Read the model definition and answer for the solid it produces. Units are mm, in the model's axes. A direction names the side the tool comes from. Coordinates: 2 decimals unless noted, no trailing zeros. Loops run counter-clockwise (first coordinate to the right, second up) from the corner with the lowest first, then second, coordinate; pieces in that order, holes last. Notation, with made-up numbers: M -30,55 L 9,55 A22 ccw 9,81 Z; hole C 21.5,41.25 d7. An arc over 180 degrees is marked long. One line per item, written item: value. Start each with the question number.
1. Flat-ended cylindrical pins translate along their axes: pin 1 (18.5 mm diameter, centred on x = 53.975, y = 0, fed in from -Z); pin 2 (1.3 mm diameter, centred on x = 16.5, z = 11.5, fed in from +Y); pin 3 (1.5 mm diameter, centred on x = 14.5, z = 6.5, fed in from -Y); pin 4 (2 mm diameter, centred on x = 15, z = 27.5, fed in from -Y). Find the tip coordinate at first contact, or state that the pin passes through.
2. The part is cut by section B-B (x = 55). Write down the section's boundary in (y, z), then the cut area to 3 significant figures.
3. Consider probe 1 along Y at (x, z) = (0, 22) (1 decimal); probe 2 along X at (y, z) = (0, 29) (1 decimal); probe 3 along Z at (x, y) = (43.5, 9.5). Determine where each line is inside the solid, lowest interval first.
4. Determine the mould class of faces 3 (the face through (22, 0, 0)), 4 (the face through (73.02, -0.42, 7.78)), 5 (the face through (-14.277, -0.559, 19.835)), 6 (the face through (-28.547, 1.256, 22.311)) for opening direction X: +X half, -X half, draft (parallel to the pull), parting line (faces both ways), or undercut.
5. The part is cut by section A-A (z = 10). State how many separate pieces and enclosed holes the cut face has, then the cut area to 3 significant figures.
6. For faces 1 (the face through (16, 4.826, 20)), 2 (the face through (29.252, -23.636, 7.776)), determine the directions among +Z, -Z, +X, -X, +Y, -Y from which every point of the face is accessible in a straight line to the end or side of a thin tool.
```python
from build123d import *

# Parameters (mm, degrees)
F0_R     = 10.16
F1_DEPTH = 15.7734
F3_DEPTH = 40.2336
F4_R     = 3.302


with BuildPart() as f1:
    # F0 (on Top) → F1 (new body)
    with BuildSketch(Plane.XY):
        with BuildLine():
            ThreePointArc((5.2118165849, 28.0956863751), (21.9710978778, 18.270234893), (28.575, 0))
            ThreePointArc((28.575, 0), (21.9710977085, -18.2702350965), (5.2118160642, -28.0956864716))
            Line((5.2118160642, -28.0956864716), (53.975, -19.05))
            ThreePointArc((53.975, -19.05), (34.925, 0), (53.975, 19.05))
            Line((53.975, 19.05), (5.2118165849, 28.0956863751))
        make_face()
        with BuildLine():
            ThreePointArc((73.025, 0), (67.4453841816, 13.4703841816), (53.975, 19.05))
            ThreePointArc((53.975, 19.05), (34.925, 0), (53.975, -19.05))
            ThreePointArc((53.975, -19.05), (67.4453841816, -13.4703841816), (73.025, 0))
        make_face()
        with Locations((53.975, 0)):
            Circle(F0_R, mode=Mode.SUBTRACT)
    extrude(amount=F1_DEPTH)

    # F2 (on face) → F3 (join)
    with BuildSketch(Plane.XY):
        with BuildLine():
            ThreePointArc((5.2118165849, 28.0956863751), (-28.575, 2.648e-07), (5.2118160642, -28.0956864716))
            ThreePointArc((5.2118160642, -28.0956864716), (21.9710977085, -18.2702350965), (28.575, 0))
            ThreePointArc((28.575, 0), (21.9710978778, 18.270234893), (5.2118165849, 28.0956863751))
        make_face()
        with BuildLine():
            Line((17.6895648793, -4.826), (13.4477648793, -4.826))
            ThreePointArc((13.4477648793, -4.826), (-14.2875, 0), (13.4477648793, 4.826))
            Line((13.4477648793, 4.826), (17.6895648793, 4.826))
            Line((17.6895648793, 4.826), (17.6895648793, -4.826))
        make_face(mode=Mode.SUBTRACT)
    extrude(amount=F3_DEPTH)

    # F4
    f4_edges = [f1.edges().sort_by_distance(p)[0] for p in [
        (-5.211816, 28.095686, 40.2336),
    ]]
    fillet(f4_edges, radius=F4_R)


solid = f1.part
```
Answer block:
1. pin 1: passes through
1. pin 2: stops at y = 26.12
1. pin 3: stops at y = -26.51
1. pin 4: stops at y = -24.91
2. outline: M -19.02,0 L -10.11,0 L -10.11,15.77 L -19.02,15.77 Z; M 10.11,0 L 19.02,0 L 19.02,15.77 L 10.11,15.77 Z
2. area: 281 mm2
3. probe 1: y = -28.6 to -14.3, 14.3 to 28.6
3. probe 2: x = -28.6 to -14.3, 17.7 to 28.6
3. probe 3: z = 0 to 15.77
4. face 3: draft
4. face 4: +X half
4. face 5: undercut
4. face 6: parting line
5. separate pieces: 1
5. enclosed holes: 2
5. area: 3,450 mm2
6. face 1: +Z, -Z
6. face 2: +Z, -Z, +X, -Y
